```python
from build123d import *

# Parameters (mm, degrees)
F1_DEPTH = 100
F2_W     = 40.5296184123
F2_H     = 20.1131775975
F3_DEPTH = 100
F4_DEPTH = 100


with BuildPart() as f1:
    # F0 (on Front) → F1 (new body)
    with BuildSketch(Plane.XZ):
        Polygon((0, 150), (0, 0), (100, 0), (100, 20), (60, 150), (40, 150), (40, 130), (20, 130), (20, 150), align=None)
    extrude(amount=F1_DEPTH)

    # F2 (on face) → F3 (cut)
    with BuildSketch(Plane(origin=(0, 0, 0), x_dir=(1, 0, 0), z_dir=(0, 0, -1))):
        with Locations((79.7351907939, 50.2432435751)):
            Rectangle(F2_W, F2_H)
    extrude(amount=-F3_DEPTH, mode=Mode.SUBTRACT)

    # F4 (cut): a face of the model
    f4_faces = [f1.faces().sort_by_distance(p)[0] for p in [
        (67.4274984862, -50.2432435751, 100),
    ]]
    extrude(f4_faces, amount=-F4_DEPTH, mode=Mode.SUBTRACT)


solid = f1.part
```
For this review, take the finished solid that the model builds, in its own axes (mm). A direction names the side the tool comes from. Give positions to 0.01 mm unless a question says otherwise; leave off trailing zeros. Loops run counter-clockwise (first coordinate to the right, second up) from the corner with the lowest first, then second, coordinate; pieces in that order, holes last. Notation, with made-up numbers: M -14.5,43.25 L 12.5,43.25 A18 ccw 12.5,52.25 Z; hole C 38,3 d9. An arc over 180 degrees is marked long. One line per item, written item: value. Start each with the question number.
Q1. Add section B-B (z = 133). Give the boundary of the cut face in (x, y), and give its area (3 significant figures).
Q2. Machinability: for faces 1 (the face through (75, -40.187, 57)), 2 (the face through (20, -49, 140)), 3 (the face through (0, -49, 76)), which of the approach directions +Z, -Z, +X, -X, +Y, -Y give a long, thin tool a straight path to every point of the face, cutting with its end or side? Answer none if there is none.
Q3. Draft analysis for pull direction Y (two halves, no side actions). For faces 4 (the face through (59.47, -50, 74)), 5 (the face through (50, -49, 150)), 6 (the face through (38, -100, 76)), state which applies: released by +Y, released by -Y, zero draft, split by the parting line, or undercut.
Q4. Clearance check with flat-ended pins moving along their axes: pin 1 Ø12 at (y, z) = (-25, 36.5) entering from +X; pin 2 Ø22 at (y, z) = (-34, 138) entering from +X; pin 3 Ø6 at (y, z) = (-48, 71) entering from +X. State where each tip first meets the part, or that it passes through.
Q5. Add section D-D (z = 16.5). Give the boundary of the cut face in (x, y), and give its area (3 significant figures).
Q6. For L1, parallel to Y at x = 82, z = 18.5; L2, parallel to Z at x = 33, y = -5; L3, parallel to X at y = -26.5, z = 141, list the stretches that pass through material, from the lowest coordinate up.
Q7. Add section C-C (y = -57). Give the boundary of the cut face in (x, z), and give its area (3 significant figures).
Q8. Add section A-A (x = 90). Give the boundary of the cut face in (y, z).
Reply:
1. outline: M 0,-100 L 20,-100 L 20,0 L 0,0 Z; M 40,-100 L 65.23,-100 L 65.23,-60.3 L 59.47,-60.3 L 59.47,-40.19 L 65.23,-40.19 L 65.23,0 L 40,0 Z
1. area: 4,410 mm²
2. face 1: +Z, -Z, +X
2. face 2: +Z, +Y, -Y
2. face 3: +Z, -Z, -X, +Y, -Y
3. face 4: undercut
3. face 5: zero draft
3. face 6: released by -Y
4. pin 1: x = 96.77
4. pin 2: x = 67.08
4. pin 3: x = 59.47
5. outline: M 0,-100 L 100,-100 L 100,-60.3 L 59.47,-60.3 L 59.47,-40.19 L 100,-40.19 L 100,0 L 0,0 Z
5. area: 9,180 mm²
6. L1: -100 to -60.3, -40.19 to 0
6. L2: 0 to 130
6. L3: 0 to 20, 40 to 62.77
7. outline: M 0,0 L 59.47,0 L 59.47,150 L 40,150 L 40,130 L 20,130 L 20,150 L 0,150 Z
7. area: 8,520 mm²
8. outline: M -100,0 L -60.3,0 L -60.3,52.5 L -100,52.5 Z; M -40.19,0 L 0,0 L 0,52.5 L -40.19,52.5 Z
